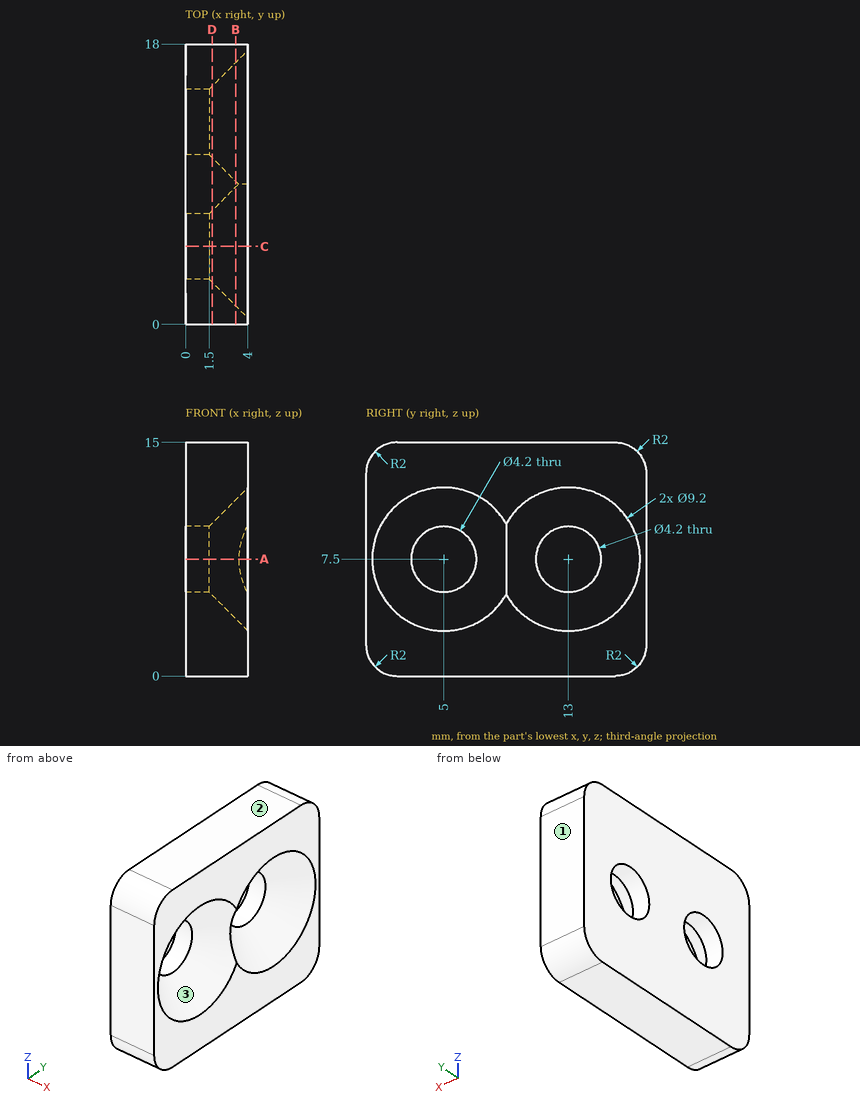
Answer from the drawing. Dimensions are ordinates in mm from the lowest x, y and z of the part. Give positions to 0.01 mm unless a question says otherwise; leave off trailing zeros. Write each loop counter-clockwise with the first axis right and the second up, starting at its lowest first coordinate (ties: lowest second). Pieces come first, ordered by that corner, then holes. Notation, with made-up numbers: (57.25, 31.5) - (74.25, 31.5) arc R27 cw to (74.25, 70.5) - close; hole circle Ø3 at (-16, 1). An arc over 180 degrees is marked (long way). Answer in a Markdown table with one row per item. Add a question column.
Item 1: Section B-B, the plane x = 3.2 is taken. Write down the section's boundary in (y, z), and give its area (3 significant figures).
Item 2: Determine the mould class of the marked faces 1, 2 and 3 for opening direction Y: pulls with the +Y half, pulls with the -Y half, needs draft (parallel to the pull), parting line crosses it, or undercut.
Item 3: Flat-ended cylindrical pins translate along their axes: P1, Ø2.5, axis at y = 13, z = 7.5, coming from the +X side; P2, Ø6.5, axis at y = 5, z = 7.5, coming from the +X side. Find the tip coordinate at first contact, or state that the pin passes through.
Item 4: Section A-A, the plane z = 7.5 is taken. Write down the section's boundary in (x, y), and give its area (3 significant figures).
Item 5: Find the intervals of material crossed by L1, parallel to Y at x = 1.25, z = 7.5; L2, parallel to Y at x = 3, z = 7.25; L3, parallel to Z at x = 3.35, y = 6.5, in increasing order.
Item 6: Section D-D, the plane x = 1.7 is taken. Write down the section's boundary in (y, z).
Item 7: Section C-C, the plane y = 5 is taken. Write down the section's boundary in (x, z).
Recorded:
| question | item | result |
|---|---|---|
| 1 | outline | (0, 2) arc R2 ccw to (2, 0) - (16, 0) arc R2 ccw to (18, 2) - (18, 13) arc R2 ccw to (16, 15) - (2, 15) arc R2 ccw to (0, 13) - close; hole circle Ø7.6 at (5, 7.5); hole circle Ø7.6 at (13, 7.5) |
| 1 | area | 176 mm2 |
| 2 | face 1 | pulls with the +Y half |
| 2 | face 2 | needs draft |
| 2 | face 3 | undercut |
| 3 | P1 | passes through |
| 3 | P2 | stops at x = 2.65 |
| 4 | outline | (0, 0) - (4, 0) - (4, 0.4) - (1.5, 2.9) - (0, 2.9) - close; (0, 7.1) - (1.5, 7.1) - (3.4, 9) - (1.5, 10.9) - (0, 10.9) - close; (0, 15.1) - (1.5, 15.1) - (4, 17.6) - (4, 18) - (0, 18) - close |
| 4 | area | 26.3 mm2 |
| 5 | L1 | y = 0 to 2.9, 7.1 to 10.9, 15.1 to 18 |
| 5 | L2 | y = 0 to 1.41, 8.59 to 9.41, 16.59 to 18 |
| 5 | L3 | z = 0 to 3.85, 11.15 to 15 |
| 6 | outline | (0, 2) arc R2 ccw to (2, 0) - (16, 0) arc R2 ccw to (18, 2) - (18, 13) arc R2 ccw to (16, 15) - (2, 15) arc R2 ccw to (0, 13) - close; hole circle Ø4.6 at (5, 7.5); hole circle Ø4.6 at (13, 7.5) |
| 7 | outline | (0, 0) - (4, 0) - (4, 2.9) - (1.5, 5.4) - (0, 5.4) - close; (0, 9.6) - (1.5, 9.6) - (4, 12.1) - (4, 15) - (0, 15) - close |
